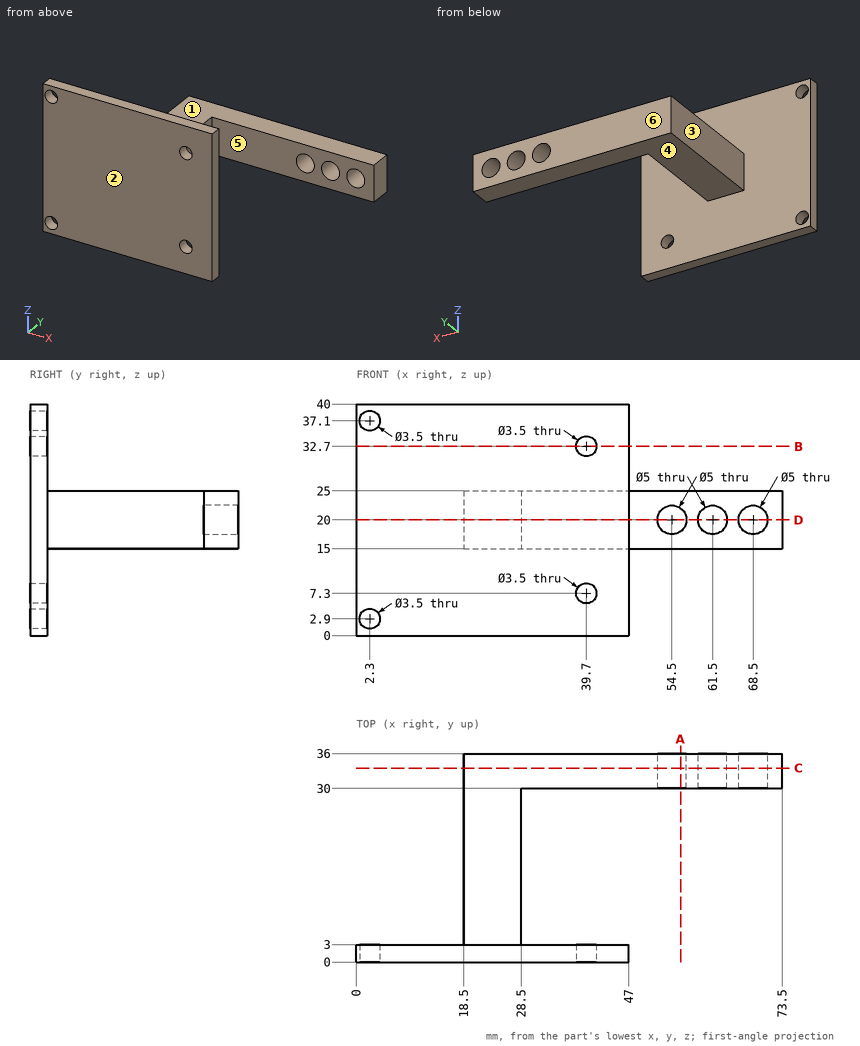
Here's the drawing with two shaded views (mm, measured from the low corner). I have some questions. A direction names the side the tool comes from. Round coordinates to 2 decimals unless told otherwise and drop trailing zeros. Loops run counter-clockwise (first coordinate to the right, second up) from the corner with the lowest first, then second, coordinate; pieces in that order, holes last. Notation, with made-up numbers: (-28.75, 70) - (-15.75, 70) arc R36 ccw to (-15.75, 105) - close; hole circle Ø5 at (-17.5, 25). An arc over 180 degrees is marked (long way). Use CSV: the item, a comma, the result in double quotes.
Item 1: If we section it at A-A on x = 56: List the corners of the cut face in (y, z) for me, then the cut area to 3 significant figures.
Here are the results:
outline,"(30, 15) - (36, 15) - (36, 18) - (30, 18) - close; (30, 22) - (36, 22) - (36, 25) - (30, 25) - close"
area,"36.0 mm²"
Item 2: If we section it at C-C on y = 33.5: List the corners of the cut face in (x, z) for me, then the cut area to 3 significant figures.
Here are the results:
outline,"(18.5, 15) - (73.5, 15) - (73.5, 25) - (18.5, 25) - close; hole circle Ø5 at (54.5, 20); hole circle Ø5 at (61.5, 20); hole circle Ø5 at (68.5, 20)"
area,"491 mm²"
Item 3: For the marked faces 1, 2 and 3, which set-ups out of +Z, -Z, +X, -X, +Y, -Y let a thin tool reach every point of the face, with its end or its side?
Here are the results:
face 1,"+Z, +X, -X, +Y"
face 2,"+Z, -Z, +X, -X, -Y"
face 3,"+Z, -Z, -X, +Y"
Item 4: Will these pins go through, and if not, where does the flat tip stop? pin 1 (6 mm diameter, centred on x = 23.5, y = 6.5, fed in from +Z); pin 2 (3 mm diameter, centred on x = 54.5, z = 20, fed in from -Y); pin 3 (5.5 mm diameter, centred on x = 2.3, z = 2.9, fed in from +Y); pin 4 (11 mm diameter, centred on y = 11.5, z = 18, fed in from +X).
Here are the results:
pin 1,"stops at z = 25"
pin 2,"passes through"
pin 3,"stops at y = 3"
pin 4,"stops at x = 28.5"
Item 5: If we section it at B-B on z = 32.7: List the corners of the cut face in (x, y) for me.
Here are the results:
outline,"(0, 0) - (37.95, 0) - (37.95, 3) - (0, 3) - close; (41.45, 0) - (47, 0) - (47, 3) - (41.45, 3) - close"
Item 6: If we mould it in two halves opening along Y, with no side actions, what happens to the marked faces 4, 5 and 6? For each: pulls with the +Y half, pulls with the -Y half, needs draft (parallel to the pull), parting line crosses it, or undercut.
Here are the results:
face 4,"needs draft"
face 5,"undercut"
face 6,"pulls with the +Y half"
Item 7: If we section it at D-D on z = 20: List the corners of the cut face in (x, y) for me.
Here are the results:
outline,"(0, 0) - (47, 0) - (47, 3) - (28.5, 3) - (28.5, 30) - (52, 30) - (52, 36) - (18.5, 36) - (18.5, 3) - (0, 3) - close; (57, 30) - (59, 30) - (59, 36) - (57, 36) - close; (64, 30) - (66, 30) - (66, 36) - (64, 36) - close; (71, 30) - (73.5, 30) - (73.5, 36) - (71, 36) - close"
Item 8: I need wall thicknesses on L1, parallel to Y at x = 45, z = 21; L2, parallel to X at y = 33.6, z = 20; L3, parallel to Z at x = 39, y = 2. Which ranges of each line are inside material? Lowest first, please. Write a range as [from, to].
Here are the results:
L1,"y = [0, 3], [30, 36]"
L2,"x = [18.5, 52], [57, 59], [64, 66], [71, 73.5]"
L3,"z = [0, 5.7], [8.9, 31.1], [34.3, 40]"
